from build123d import *
from build123d.topology import SkipClean

# Parameters (mm, degrees)
BOSS_EXTRUDE1_DEPTH             = 25
BOSS_EXTRUDE2_REACH             = 65.436
BOSS_EXTRUDE2_DIRECTION_2_DEPTH = 30
SKETCH9_R                       = 2.05
CUT_EXTRUDE3_DEPTH              = 35.1
BOSS_EXTRUDE5_REACH             = 63.632
SKETCH13_R                      = 1.55
CUT_EXTRUDE4_DEPTH              = 88.768186926
SKETCH16_W                      = 63
SKETCH16_H                      = 45
CUT_EXTRUDE5_DEPTH              = 65.271143


with BuildPart() as part:
    # Sketch1 → Boss-Extrude1 (new, symmetric)
    with BuildSketch(Plane.XY):
        with BuildLine():
            Line((-17.55, 22.5), (-17.55, 0))
            Line((-17.55, 0), (17.55, 0))
            Line((17.55, 0), (17.55, 22.5))
            Line((17.55, 22.5), (12.55, 22.5))
            ThreePointArc((12.55, 22.5), (0, 9.95), (-12.55, 22.5))
            Line((-12.55, 22.5), (-17.55, 22.5))
        make_face()
    boss_extrude1 = extrude(amount=BOSS_EXTRUDE1_DEPTH, both=True)

    # Boss-Extrude2: up to this face of the body (flat: up to its plane)
    boss_extrude2_end = Plane(part.part.faces().sort_by_distance((17.55, 11.25, 0))[0])
    # Sketch5 → Boss-Extrude2 (add, up to the picked face)
    with BuildSketch(Plane(origin=(26.152881057, 0, 15.099372918), x_dir=(0.500000000000001, 0, -0.8660254037844382), z_dir=(0.8660254037844382, 0, 0.500000000000001)), mode=Mode.PRIVATE) as boss_extrude2_sk1:
        with BuildLine():
            Line((-8.725, 22.5), (-3.775, 22.5))
            ThreePointArc((-3.775, 22.5), (8.775, 9.95), (21.325, 22.5))
            Line((21.325, 22.5), (26.275, 22.5))
            ThreePointArc((26.275, 22.5), (8.775, 5), (-8.725, 22.5))
        make_face()
    boss_extrude2_tool1 = split(extrude(boss_extrude2_sk1.sketch, amount=-BOSS_EXTRUDE2_REACH, mode=Mode.PRIVATE), bisect_by=boss_extrude2_end, keep=Keep.BOTH, mode=Mode.PRIVATE)
    boss_extrude2 = boss_extrude2_tool1.solids().sort_by(Axis((23.027881, 22.108688, 20.512032), (-0.8660254037844382, 0, -0.500000000000001)))[0]
    add(boss_extrude2)

    # Sketch5 → Boss-Extrude2 direction 2 (add)
    with BuildSketch(Plane(origin=(26.152881057, 0, 15.099372918), x_dir=(0.500000000000001, 0, -0.8660254037844382), z_dir=(0.8660254037844382, 0, 0.500000000000001))):
        with BuildLine():
            Line((-8.725, 22.5), (-3.775, 22.5))
            ThreePointArc((-3.775, 22.5), (8.775, 9.95), (21.325, 22.5))
            Line((21.325, 22.5), (26.275, 22.5))
            ThreePointArc((26.275, 22.5), (8.775, 5), (-8.725, 22.5))
        make_face()
    boss_extrude2_direction_2 = extrude(amount=BOSS_EXTRUDE2_DIRECTION_2_DEPTH)

    # Sketch9 → Cut-Extrude3 (cut)
    with BuildSketch(Plane.ZY.offset(17.55)):
        with Locations((-18, 5)):
            Circle(SKETCH9_R)
        with Locations((18, 5)):
            Circle(SKETCH9_R)
    cut_extrude3 = extrude(amount=-CUT_EXTRUDE3_DEPTH, mode=Mode.SUBTRACT)

    # Boss-Extrude5: up to this face of the body (flat: up to its plane)
    boss_extrude5_end = Plane(part.part.faces().sort_by_distance((17.55, 17.173614571, 0))[0])
    # Sketch12 → Boss-Extrude5 (add, up to the picked face)
    with BuildSketch(Plane(origin=(22.035576211, 0, 12.722245857), x_dir=(0.4999999999999999, 0, -0.8660254037844388), z_dir=(0.8660254037844388, 0, 0.4999999999999999)), mode=Mode.PRIVATE) as boss_extrude5_sk1:
        with BuildLine():
            Line((-3.775, 22.5), (21.325, 22.5))
            ThreePointArc((21.325, 22.5), (8.775, 9.95), (-3.775, 22.5))
        make_face()
    boss_extrude5_tool1 = split(extrude(boss_extrude5_sk1.sketch, amount=-BOSS_EXTRUDE5_REACH, mode=Mode.PRIVATE), bisect_by=boss_extrude5_end, keep=Keep.BOTH, mode=Mode.PRIVATE)
    boss_extrude5 = boss_extrude5_tool1.solids().sort_by(Axis((26.423076, 17.173615, 5.122873), (-0.8660254037844388, 0, -0.4999999999999999)))[0]
    add(boss_extrude5)


with BuildPart() as mirror1_1:
    # Mirror1: Boss-Extrude1, Boss-Extrude2, Boss-Extrude2 direction 2 across plane
    add(boss_extrude1.mirror(Plane(origin=(17.55, 22.5, 25), x_dir=(0, 0, 1), z_dir=(0, -1, 0))))
    add(boss_extrude2.mirror(Plane(origin=(17.55, 22.5, 25), x_dir=(0, 0, 1), z_dir=(0, -1, 0))))
    add(boss_extrude2_direction_2.mirror(Plane(origin=(17.55, 22.5, 25), x_dir=(0, 0, 1), z_dir=(0, -1, 0))))

    # Mirror1 2: Cut-Extrude3 across plane
    add(cut_extrude3.mirror(Plane(origin=(17.55, 22.5, 25), x_dir=(0, 0, 1), z_dir=(0, -1, 0))), mode=Mode.SUBTRACT)


with BuildPart() as mirror1_3_1:
    # Mirror1 3: Boss-Extrude5 across plane
    add(boss_extrude5.mirror(Plane(origin=(17.55, 22.5, 25), x_dir=(0, 0, 1), z_dir=(0, -1, 0))))


with BuildPart() as part_1:
    add(part.part)

    # Mirror1 united with what the copies touc: union Mirror1_1, Mirror1 3_1
    add(mirror1_1.part)
    add(mirror1_3_1.part)

    # Sketch13 → Cut-Extrude4 (cut, through all)
    with SkipClean():  # the faces are left unmerged after this step: merging them gives an invalid solid
        with BuildSketch(Plane(origin=(0, 0, 0), x_dir=(1, 0, 0), z_dir=(0, 1, 0))):
            with Locations(Location((43.530762114, -15, 0), (0, 0, 90))):
                Circle(SKETCH13_R)
        extrude(amount=CUT_EXTRUDE4_DEPTH, mode=Mode.SUBTRACT)

    # Sketch16 → Cut-Extrude5 (cut)
    with BuildSketch(Plane(origin=(0, 0, 0), x_dir=(0, 0, -1), z_dir=(1, 0, 0))):
        with Locations((-6.5, 22.5)):
            Rectangle(SKETCH16_W, SKETCH16_H)
    extrude(amount=CUT_EXTRUDE5_DEPTH, mode=Mode.SUBTRACT)


solid = part_1.part
Build history of the part. All positions in model axes, mm. Round coordinates to 2 decimals unless told otherwise and drop trailing zeros. Loops run counter-clockwise (first coordinate to the right, second up) from the corner with the lowest first, then second, coordinate; pieces in that order, holes last. Notation, with made-up numbers: (-20, -31) -> (6, -31) arc R10 cw to (6, -13) -> close; hole circle Ø1 at (42, 6.5). An arc over 180 degrees is marked (long way). One line per item, written item: value. Start each with the question number.
Q1. Probe line 1 along Z through (x, y) = (-7.5, 40); line 2 along Z through (x, y) = (-14.5, 4); line 3 along Y through (x, z) = (-10.5, -18). List the from-to ranges inside material, lowest first.
Q2. Cut at D-D on x = -7.25. List the corners of the cut face in (y, z), plus the area to 3 significant figures.
Q3. Cut at C-C on x = -1.5. List the corners of the cut face in (y, z), plus the area to 3 significant figures.
Q4. Drop a flat-ended pin along its axis: pin 1 Ø1 at (y, z) = (16.5, 16) entering from +X. Give the stop position or say it passes through.
Q5. Cut at B-B on y = 40. List the corners of the cut face in (x, z).
Q6. Two-plate mould, pull along Y, no slides. Class faces 1 (the face through (0, 40, 0)), 2 (the face through (-8.898, 37.967, -18.267)), 3 (the face through (-9, 0, 0)): released by +Y, released by -Y, zero draft, split by the parting line, or undercut.
Q7. Cut at A-A on z = 18. List the corners of the cut face in (x, y), plus the area to 3 significant figures.
Computed:
1. line 1: -25 to -20.05, -15.95 to 15.95, 20.05 to 25
1. line 2: -25 to -19.79, -16.21 to 16.21, 19.79 to 25
1. line 3: 0 to 2.95, 7.05 to 15.63, 29.37 to 37.95, 42.05 to 45
2. outline: (0, -25) -> (12.26, -25) -> (12.26, 25) -> (0, 25) -> close; (32.74, -25) -> (45, -25) -> (45, 25) -> (32.74, 25) -> close; hole circle Ø4.1 at (5, -18); hole circle Ø4.1 at (5, 18); hole circle Ø4.1 at (40, -18); hole circle Ø4.1 at (40, 18)
2. area: 1,170 mm²
3. outline: (0, -25) -> (10.04, -25) -> (10.04, 25) -> (0, 25) -> close; (34.96, -25) -> (45, -25) -> (45, 25) -> (34.96, 25) -> close; hole circle Ø4.1 at (5, -18); hole circle Ø4.1 at (5, 18); hole circle Ø4.1 at (40, -18); hole circle Ø4.1 at (40, 18)
3. area: 951 mm²
4. pin 1: x = -10.74
5. outline: (-17.55, -25) -> (0, -25) -> (0, -20.05) -> (-17.55, -20.05) -> close; (-17.55, -15.95) -> (0, -15.95) -> (0, 15.95) -> (-17.55, 15.95) -> close; (-17.55, 20.05) -> (0, 20.05) -> (0, 25) -> (-17.55, 25) -> close
6. face 1: zero draft
6. face 2: undercut
6. face 3: released by -Y
7. outline: (-17.55, 0) -> (0, 0) -> (0, 2.95) -> (-17.55, 2.95) -> close; (-17.55, 7.05) -> (0, 7.05) -> (0, 9.95) arc R12.55 cw to (0, 35.05) -> (0, 37.95) -> (-17.55, 37.95) -> close; (-17.55, 42.05) -> (0, 42.05) -> (0, 45) -> (-17.55, 45) -> close
7. area: 398 mm²
